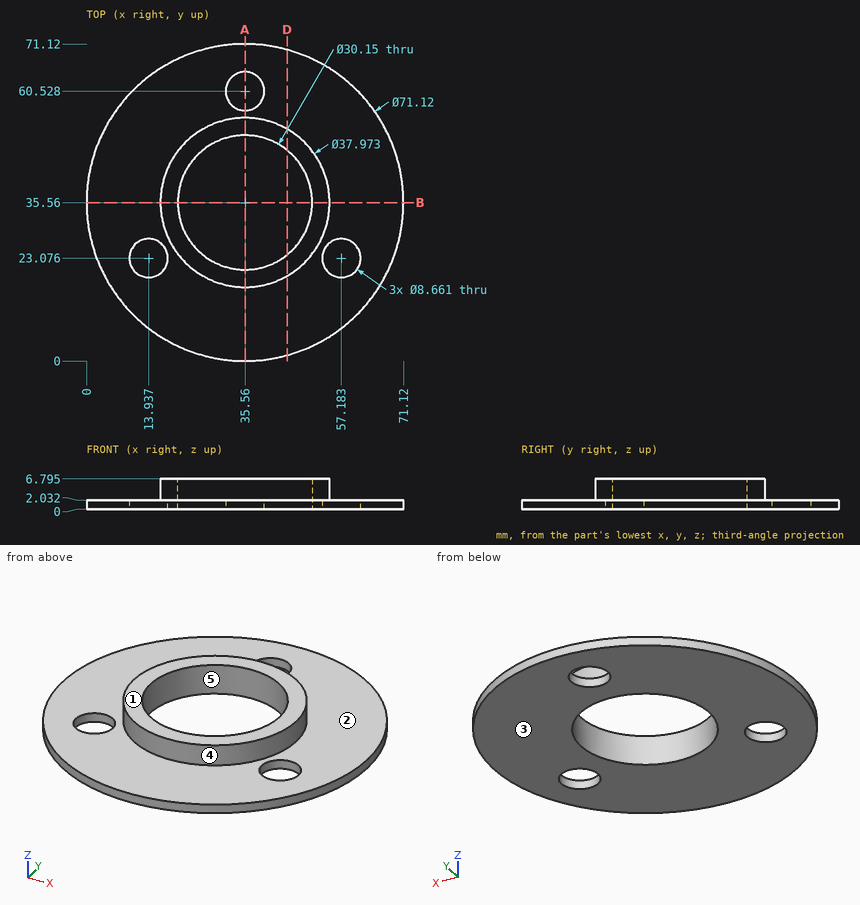
Study the drawing (mm; zero at the part's minimum x, y, z) and answer. A direction names the side the tool comes from. Round coordinates to 2 decimals unless told otherwise and drop trailing zeros. Write each loop counter-clockwise with the first axis right and the second up, starting at its lowest first coordinate (ties: lowest second). Pieces come first, ordered by that corner, then holes.
1) A cutting plane is placed at B-B on y = 35.56. Determine the outline of the cut face in (x, z) (1 decimal).
2) Determine the mould class of the marked faces 3, 4 and 5 for opening direction Y: pulls with the +Y half, pulls with the -Y half, needs draft (parallel to the pull), parting line crosses it, or undercut.
3) Which of the six approach directions +Z, -Z, +X, -X, +Y, -Y give full straight-line access (tool end or side, diameter ignored) to the marked faces 1 and 2?
4) Flat-ended cylindrical pins translate along their axes: P1, Ø3, axis at x = 20.5, y = 12.5, coming from the +Z side; P2, Ø4, axis at y = 39, z = 1.5, coming from the -X side; P3, Ø1.5, axis at y = 56, z = 3.5, coming from the +X side; P4, Ø1.5, axis at y = 34, z = 4.5, coming from the -X side. Find the tip coordinate at first contact, or state that the pin passes through.
5) Consider probe 1 along Y at (x, z) = (35.56, 0.55) (1 decimal); probe 2 along Y at (x, z) = (35.56, 3) (1 decimal); probe 3 along Z at (x, y) = (8, 13.5). Determine where each line is inside the solid, lowest interval first.
6) A cutting plane is placed at A-A on x = 35.56. Determine the outline of the cut face in (y, z) (1 decimal).
7) A cutting plane is placed at D-D on x = 45. Determine the outline of the cut face in (y, z) (1 decimal).
Entries:
1. outline: (0, 0) - (20.5, 0) - (20.5, 6.8) - (16.6, 6.8) - (16.6, 2) - (0, 2) - close; (50.6, 0) - (71.1, 0) - (71.1, 2) - (54.5, 2) - (54.5, 6.8) - (50.6, 6.8) - close
2. face 3: needs draft
2. face 4: parting line crosses it
2. face 5: undercut
3. face 1: +Z, +X, -X, +Y, -Y
3. face 2: +Z
4. P1: stops at z = 2.03
4. P2: stops at x = 0.03
4. P3: passes through
4. P4: stops at x = 16.59
5. probe 1: y = 0 to 20.5, 50.6 to 56.2, 64.9 to 71.1
5. probe 2: y = 16.6 to 20.5, 50.6 to 54.5
5. probe 3: z = 0 to 2.03
6. outline: (0, 0) - (20.5, 0) - (20.5, 6.8) - (16.6, 6.8) - (16.6, 2) - (0, 2) - close; (50.6, 0) - (56.2, 0) - (56.2, 2) - (54.5, 2) - (54.5, 6.8) - (50.6, 6.8) - close; (64.9, 0) - (71.1, 0) - (71.1, 2) - (64.9, 2) - close
7. outline: (1.3, 0) - (23.8, 0) - (23.8, 6.8) - (19.1, 6.8) - (19.1, 2) - (1.3, 2) - close; (47.3, 0) - (69.8, 0) - (69.8, 2) - (52, 2) - (52, 6.8) - (47.3, 6.8) - close
